from build123d import *

# Parameters (mm, degrees)
SKIZZE1_R                        = 22.5
SEITE1_DEPTH                     = 2
SKIZZE2_R                        = 20.5
LAUFFL_CHE_DEPTH                 = 8
SKIZZE5_R                        = 22.5
SEITE_2_DEPTH                    = 2
BOHRUNG_DEPTH                    = 100
BOHRUNG_DEPTH_BACK               = 34.35416016
SKIZZE7_R                        = 2.5
SKIZZE9_R                        = 10
ZAPFEN_DEPTH                     = 37
F_12_0_12_DURCHMESSER_BOHRUNG1_D = 12


with BuildPart() as part:
    # Skizze1 → Seite1 (new body)
    with BuildSketch(Plane.XY):
        Circle(SKIZZE1_R)
    extrude(amount=SEITE1_DEPTH)

    # Skizze2 → Lauffläche (add)
    with BuildSketch(Plane.XY):
        Circle(SKIZZE2_R)
    extrude(amount=LAUFFL_CHE_DEPTH)

    # Skizze5 → Seite 2 (add)
    with BuildSketch(Plane.XY.offset(8)):
        Circle(SKIZZE5_R)
    extrude(amount=SEITE_2_DEPTH)

    # Skizze7 → Bohrung (cut, two sides: drawn at the far end of the back side and taken through both)
    with BuildSketch(Plane.XY.offset(-BOHRUNG_DEPTH_BACK)):
        Circle(SKIZZE7_R)
    extrude(amount=BOHRUNG_DEPTH + BOHRUNG_DEPTH_BACK, mode=Mode.SUBTRACT)

    # Skizze9 → Zapfen (add)
    with BuildSketch(Plane.XY.offset(10)):
        Circle(SKIZZE9_R)
    extrude(amount=ZAPFEN_DEPTH)

    # Ø12.0 (12) Durchmesser Bohrung1 (through all)
    with Locations(Plane(origin=(0, 0, 0), x_dir=(-1, 0, 0), z_dir=(0, 0, -1))):
        with Locations((0, 0)):
            Hole(F_12_0_12_DURCHMESSER_BOHRUNG1_D / 2)


solid = part.part
Source: CAD feature listing. Evaluate the final solid. Frame: model axes, mm. A direction names the side the tool comes from. Give positions to 0.01 mm unless a question says otherwise; leave off trailing zeros. Loops run counter-clockwise (first coordinate to the right, second up) from the corner with the lowest first, then second, coordinate; pieces in that order, holes last. Notation, with made-up numbers: (27, 72.25) -> (60, 72.25) arc R9 cw to (60, 88.25) -> close; hole circle Ø2 at (57.25, 54.5). An arc over 180 degrees is marked (long way). Use a Markdown table: item, result. Add a question column.
1) First-contact query: pin 1 (13.5 mm diameter, centred on x = 7, y = -6.5, fed in from -Z); pin 2 (3 mm diameter, centred on x = 10, z = 11, fed in from +Y); pin 3 (12 mm diameter, centred on x = 9, z = 33, fed in from +Y); pin 4 (6 mm diameter, centred on y = 14.5, z = 21.5, fed in from -X). Flat tips, straight axial feed; report the tip coordinate or a pass-through.
2) Reachability of faces 1 (the face through (10.382, -19.961, 8.986)), 2 (the face through (9.9, -18.2, 8)), 3 (the face through (5, -10, 10)) from +Z, -Z, +X, -X, +Y, -Y: full face, straight path, thin tool, end or side. Return the list, or none.
3) Section query A-A, the plane x = 0. Return the cut outline in (y, z).
4) Line query: line 1 along Y through (x, z) = (0, 35.5); line 2 along Z through (x, y) = (16, 8); line 3 along X through (y, z) = (1, 22). Output: solid intervals per line, ascending. Write a range as [from, to].
5) Section query D-D, the plane x = -8. Return the cut outline in (y, z).
6) Pull-direction query (Z, two-part tool) for faces 4 (the face through (9.9, -18.2, 2)), 5 (the face through (0, -7, 47)), 6 (the face through (-4.444, -20.013, 4.958)), 7 (the face through (-6, 0, 24)); classes: +Z half, -Z half, draft (parallel to the pull), parting line (faces both ways), or undercut.
7) Section query C-C, the plane z = 6. Return the cut outline in (x, y).
Numbers:
| question | item | result |
|---|---|---|
| 1 | pin 1 | stops at z = 0 |
| 1 | pin 2 | stops at y = 20.67 |
| 1 | pin 3 | stops at y = 9.54 |
| 1 | pin 4 | passes through |
| 2 | face 1 | +Z, -Z |
| 2 | face 2 | none |
| 2 | face 3 | +Z |
| 3 | outline | (-22.5, 0) -> (-6, 0) -> (-6, 47) -> (-10, 47) -> (-10, 10) -> (-22.5, 10) -> (-22.5, 8) -> (-20.5, 8) -> (-20.5, 2) -> (-22.5, 2) -> close; (6, 0) -> (22.5, 0) -> (22.5, 2) -> (20.5, 2) -> (20.5, 8) -> (22.5, 8) -> (22.5, 10) -> (10, 10) -> (10, 47) -> (6, 47) -> close |
| 4 | line 1 | y = [-10, -6], [6, 10] |
| 4 | line 2 | z = [0, 10] |
| 4 | line 3 | x = [-9.95, -5.92], [5.92, 9.95] |
| 5 | outline | (-21.03, 0) -> (21.03, 0) -> (21.03, 2) -> (18.87, 2) -> (18.87, 8) -> (21.03, 8) -> (21.03, 10) -> (6, 10) -> (6, 47) -> (-6, 47) -> (-6, 10) -> (-21.03, 10) -> (-21.03, 8) -> (-18.87, 8) -> (-18.87, 2) -> (-21.03, 2) -> close |
| 6 | face 4 | undercut |
| 6 | face 5 | +Z half |
| 6 | face 6 | undercut |
| 6 | face 7 | draft |
| 7 | outline | circle Ø41 at (0, 0); hole circle Ø12 at (0, 0) |
